CAD build for the part. Positions are in the model's coordinates, mm. Face numbers are marked on the shaded views. A direction names the side the tool comes from. Give positions to 0.01 mm unless a question says otherwise; leave off trailing zeros. Order: outer loops, then holes, each group sorted by start corner. A loop starts at its lowest first (then second) coordinate and runs counter-clockwise, first axis right, second up.
Item 1: Band-saw the part on A-A on z = 0.3. Give the cut face in (x, y) (3 decimals), plus the area to 3 significant figures.
Item 2: Which spindle directions (+Z, -Z, +X, -X, +Y, -Y) get a long thin tool onto all of the face, cutting with end or side? Do the marked faces 1 and 2. Say none if no direction does.
Item 3: Wall check: L1, parallel to Y at x = -1.5, z = 1.1; L2, parallel to Y at x = -1.25, z = 0.15; L3, parallel to X at y = -8.5, z = 0.2. Give the ranges that are in metal, low to high.
Item 4: Band-saw the part on B-B on y = -4.5. Give the cut face in (x, z), plus the area to 3 significant figures.
Item 5: Band-saw the part on D-D on y = -9.75. Give the cut face in (x, z), plus the area to 3 significant figures.
Item 6: Band-saw the part on C-C on x = -1.75. Give the cut face in (y, z).
Item 7: Flat gauge pins, fed straight in: P1, Ø0.8, axis at x = -1.78, y = -4.11, coming from the -Z side; P2, Ø0.6, axis at y = -6.5, z = 0.5, coming from the +X side. Where does each tip first touch, or does it go through?
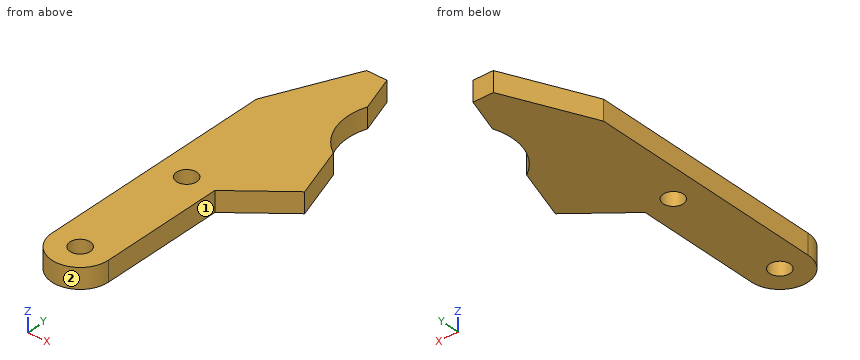
```python
from build123d import *

# Parameters (mm, degrees)
SKETCH1_R           = 0.635
BOSS_EXTRUDE1_DEPTH = 1.27


with BuildPart() as part:
    # Sketch1 → Boss-Extrude1 (new body)
    with BuildSketch(Plane.XY):
        with BuildLine():
            Line((0, -11.938), (0, -4.107900924))
            Line((0, -4.107900924), (3.332623342, -1.403875353))
            Line((3.332623342, -1.403875353), (2.227712005, 1.993118473))
            ThreePointArc((2.227712005, 1.993118473), (0.867392125, 3.796133525), (0.906732127, 6.054404062))
            Line((0.906732127, 6.054404062), (0.139174217, 8.382))
            Line((0.139174217, 8.382), (-1.138657386, 8.382))
            Line((-1.138657386, 8.382), (-3.556, 3.099290623))
            Line((-3.556, 3.099290623), (-3.556, -11.938))
            ThreePointArc((-3.556, -11.938), (-1.778, -13.716), (0, -11.938))
        make_face()
        with Locations((-1.778, -11.938)):
            Circle(SKETCH1_R, mode=Mode.SUBTRACT)
        with Locations((-1.778, -4.107900924)):
            Circle(SKETCH1_R, mode=Mode.SUBTRACT)
    extrude(amount=BOSS_EXTRUDE1_DEPTH)


solid = part.part
```
The answers:
1. outline: (-3.556, -11.938) arc R1.778 ccw to (0, -11.938) - (0, -4.108) - (3.333, -1.404) - (2.228, 1.993) arc R3.466 cw to (0.907, 6.054) - (0.139, 8.382) - (-1.139, 8.382) - (-3.556, 3.099) - close; hole circle Ø1.27 at (-1.778, -11.938); hole circle Ø1.27 at (-1.778, -4.108)
1. area: 87.7 mm2
2. face 1: +Z, -Z, +X, -Y
2. face 2: +Z, -Z, -Y
3. L1: y = -13.69 to -12.51, -11.37 to -4.68, -3.54 to 7.59
3. L2: y = -13.64 to -12.29, -11.59 to -4.46, -3.76 to 8.14
3. L3: x = -3.56 to 0
4. outline: (-3.56, 0) - (-2.28, 0) - (-2.28, 1.27) - (-3.56, 1.27) - close; (-1.28, 0) - (0, 0) - (0, 1.27) - (-1.28, 1.27) - close
4. area: 3.25 mm2
5. outline: (-3.56, 0) - (0, 0) - (0, 1.27) - (-3.56, 1.27) - close
5. area: 4.52 mm2
6. outline: (-13.72, 0) - (-12.57, 0) - (-12.57, 1.27) - (-13.72, 1.27) - close; (-11.3, 0) - (-4.74, 0) - (-4.74, 1.27) - (-11.3, 1.27) - close; (-3.47, 0) - (7.05, 0) - (7.05, 1.27) - (-3.47, 1.27) - close
7. P1: passes through
7. P2: stops at x = 0
